```python
from build123d import *

# Parameters (mm, degrees)
F0_R     = 6
F1_DEPTH = 20
F2_R     = 10
F4_D     = 8
F4_DEPTH = 10
F4_TIP   = 2.4034424761
F5_R     = 17.99999


# Not quite as in the source:
# - a fillet or chamfer is up to 0.001 mm smaller than in the source, because OpenCascade refuses the exact size


with BuildPart() as f1:
    # F0 (on Front) → F1 (new body)
    with BuildSketch(Plane.XZ):
        with BuildLine():
            Line((-20, 0), (-11.25, -9.9215674165))
            ThreePointArc((-11.25, -9.9215674165), (5.3033008589, -14.0312152004), (15, 0))
            Line((15, 0), (15, 15))
            Line((15, 15), (15, 18))
            Line((15, 18), (-65, 18))
            Line((-65, 18), (-65, 0))
            Line((-65, 0), (-20, 0))
        make_face()
        Circle(F0_R, mode=Mode.SUBTRACT)
    extrude(amount=F1_DEPTH)

    # F2
    f2_edges = [f1.edges().sort_by_distance(p)[0] for p in [
        (-20, -10, 0),
    ]]
    fillet(f2_edges, radius=F2_R)

    # F4
    with Locations(Plane.XY.offset(18)):
        with Locations((-45, -10), (-20, -10)):
            Hole(F4_D / 2, depth=F4_DEPTH)
            with Locations((0, 0, -(F4_DEPTH + F4_TIP / 2))):  # 118° drill point
                Cone(0, F4_D / 2, F4_TIP, mode=Mode.SUBTRACT)

    # F5 (radius 18 in the source; OpenCascade refuses exactly that, so slightly less here)
    f5_edges = [f1.edges().sort_by_distance(p)[0] for p in [
        (-65, -10, 0),
    ]]
    fillet(f5_edges, radius=F5_R)


solid = f1.part
```
The model under review builds one solid part; all positions refer to its coordinate system, in mm. A direction names the side the tool comes from. Round coordinates to 2 decimals unless told otherwise and drop trailing zeros. Loops run counter-clockwise (first coordinate to the right, second up) from the corner with the lowest first, then second, coordinate; pieces in that order, holes last.
Item 1: Take a section at C-C (z = 11). Write out the cut boundary in (x, y), then the cut area to 3 significant figures.
Determined:
outline: (-63.58, -20) - (15, -20) - (15, 0) - (-63.58, 0) - close; hole circle Ø8 at (-45, -10); hole circle Ø8 at (-20, -10)
area: 1,470 mm2
Item 2: Take a section at D-D (x = -40). Write out the cut boundary in (y, z).
Determined:
outline: (-20, 0) - (0, 0) - (0, 18) - (-20, 18) - close
Item 3: For line 1 (Y direction, x = -20, z = 12); line 2 (X direction, y = -10, z = 10.25); line 3 (Z direction, x = 0, y = -6.5), list the stretches that pass through material, from the lowest coordinate up.
Determined:
line 1: y = -20 to -14, -6 to 0
line 2: x = -63.25 to -49, -41 to -24, -16 to 15
line 3: z = -15 to -6, 6 to 18
Item 4: Mouldability with a two-part tool opening along X and no side actions: class faces 1 (the face through (-14.17, -9.86, -6.61)), 2 (the face through (-17, 0, 5)), 3 (the face through (-45.512, -9.531, 6.014)) as released by +X, released by -X, zero draft, split by the parting line, or undercut.
Determined:
face 1: released by -X
face 2: zero draft
face 3: undercut
Item 5: For faces 4 (the face through (-36, -10, 0)), 5 (the face through (5.06, -9.86, -14.12)), 6 (the face through (-16.8, -12.4, 12.9)), list the 3-axis set-ups (+Z, -Z, +X, -X, +Y, -Y) from which the entire face can be reached by the end or side of a thin tool; tool diameter is ignored.
Determined:
face 4: -Z, -X, +Y, -Y
face 5: -Z, +Y, -Y
face 6: +Z
Item 6: Take a section at B-B (z = 3). Write out the cut boundary in (x, y).
Determined:
outline: (-56.95, -20) - (-5.2, -20) - (-5.2, 0) - (-56.95, 0) - close; (5.2, -20) - (15, -20) - (15, 0) - (5.2, 0) - close
Item 7: Clearance check with flat-ended pins moving along their axes: pin 1 Ø10 at (x, y) = (6, -12.5) entering from -Z; pin 2 Ø5 at (y, z) = (-10.5, -11.5) entering from +X; pin 3 Ø1 at (y, z) = (-10, 14.5) entering from -X. State where each tip first meets the part, or that it passes through.
Determined:
pin 1: stops at z = -14.97
pin 2: stops at x = 12
pin 3: stops at x = -64.75
